Work out the finished part from the listing and answer in its coordinate system (mm). A direction names the side the tool comes from. Give positions to 0.01 mm unless a question says otherwise; leave off trailing zeros. Loops run counter-clockwise (first coordinate to the right, second up) from the corner with the lowest first, then second, coordinate; pieces in that order, holes last. Notation, with made-up numbers: (-25.5, -17) - (-15.5, -17) arc R24 ccw to (-15.5, 2) - close; hole circle Ø8 at (35, 4.25). An arc over 180 degrees is marked (long way). One line per item, written item: value.
from build123d import *

# Parameters (mm, degrees)
F0_R     = 12.7
F0_R_2   = 4.7625
F1_DEPTH = 12.7
F2_R     = 15.875
F2_R_2   = 4.7625
F3_DEPTH = 3.175
F4_R     = 15.875
F4_R_2   = 4.7625
F5_DEPTH = 3.175
F6_R     = 3.175
F7_DEPTH = 6.35


with BuildPart() as f1:
    # F0 (on Top) → F1 (new body)
    with BuildSketch(Plane.XY):
        Circle(F0_R)
        Circle(F0_R_2, mode=Mode.SUBTRACT)
    extrude(amount=F1_DEPTH)

    # F2 (on face) → F3 (join)
    with BuildSketch(Plane.XY.offset(12.7)):
        Circle(F2_R)
        Circle(F2_R_2, mode=Mode.SUBTRACT)
    extrude(amount=F3_DEPTH)

    # F4 (on Top) → F5 (join)
    with BuildSketch(Plane.XY):
        Circle(F4_R)
        Circle(F4_R_2, mode=Mode.SUBTRACT)
    extrude(amount=F5_DEPTH)

    # F6 (on face) → F7 (join)
    with BuildSketch(Plane(origin=(0, 0, 0), x_dir=(1, 0, 0), z_dir=(0, 0, -1))):
        with Locations((9.525, 0)):
            Circle(F6_R)
    extrude(amount=F7_DEPTH)


solid = f1.part
1. For faces 4 (the flat face through (9, 0, -6.35)), 5 (the cylindrical face through (-2.75, -12.4, 7.87)), determine the directions among +Z, -Z, +X, -X, +Y, -Y from which every point of the face is accessible in a straight line to the end or side of a thin tool.
Output:
face 4: -Z, +X, -X, +Y, -Y
face 5: none
2. Find the intervals of material crossed by line 1 along Z through (x, y) = (-3, -12.5) (3 decimals); line 2 along Y through (x, z) = (0, 9); line 3 along Z through (x, y) = (-2, 8.5) (3 decimals), in increasing order.
Output:
line 1: z = 0 to 3.175, 12.7 to 15.875
line 2: y = -12.7 to -4.76, 4.76 to 12.7
line 3: z = 0 to 15.875
3. Flat-ended cylindrical pins translate along their axes: pin 1 Ø3 at (y, z) = (0, 5.5) entering from -X; pin 2 Ø16 at (x, y) = (-1.5, -7) entering from -Z; pin 3 Ø5 at (y, z) = (-12, 13.5) entering from +X. Find the tip coordinate at first contact, or state that the pin passes through.
Output:
pin 1: stops at x = -12.7
pin 2: stops at z = 0
pin 3: stops at x = 12.72
4. Section B-B (x = 0) is taken. Write down the section's boundary in (y, z) (1 decimal), and give its area (3 significant figures).
Output:
outline: (-15.9, 0) - (-4.8, 0) - (-4.8, 15.9) - (-15.9, 15.9) - (-15.9, 12.7) - (-12.7, 12.7) - (-12.7, 3.2) - (-15.9, 3.2) - close; (4.8, 0) - (15.9, 0) - (15.9, 3.2) - (12.7, 3.2) - (12.7, 12.7) - (15.9, 12.7) - (15.9, 15.9) - (4.8, 15.9) - close
area: 292 mm²
5. Section C-C (z = 11) is taken. Write down the section's boundary in (x, y) (1 decimal), and give its area (3 significant figures).
Output:
outline: circle Ø25.4 at (0, 0); hole circle Ø9.5 at (0, 0)
area: 435 mm²
6. The mould has two halves that part along X. Classify faces 1 (the cylindrical face through (-3.78, -2.9, 7.83)), 2 (the flat face through (-4, -3, 0)), 3 (the cylindrical face through (12.458, 1.216, -3.131)): released by +X, released by -X, zero draft, split by the parting line, or undercut.
Output:
face 1: undercut
face 2: zero draft
face 3: split by the parting line
7. Section D-D (y = 10.5) is taken. Write down the section's boundary in (x, z) (3 decimals).
Output:
outline: (-11.907, 0) - (11.907, 0) - (11.907, 3.175) - (7.144, 3.175) - (7.144, 12.7) - (11.907, 12.7) - (11.907, 15.875) - (-11.907, 15.875) - (-11.907, 12.7) - (-7.144, 12.7) - (-7.144, 3.175) - (-11.907, 3.175) - close
